The drawing under review shows one solid part. Ordinate dimensions are in mm from its lowest x, y, z. A direction names the side the tool comes from. Coordinates: 2 decimals unless noted, no trailing zeros. Order: outer loops, then holes, each group sorted by start corner. A loop starts at its lowest first (then second) coordinate and runs counter-clockwise, first axis right, second up. Notation, with made-up numbers: M 41,73.5 L 92,73.5 A35 ccw 92,105.5 Z; hole C -23.5,-38.75 d8. An arc over 180 degrees is marked long. Answer as a JSON object with one key per item and string values.
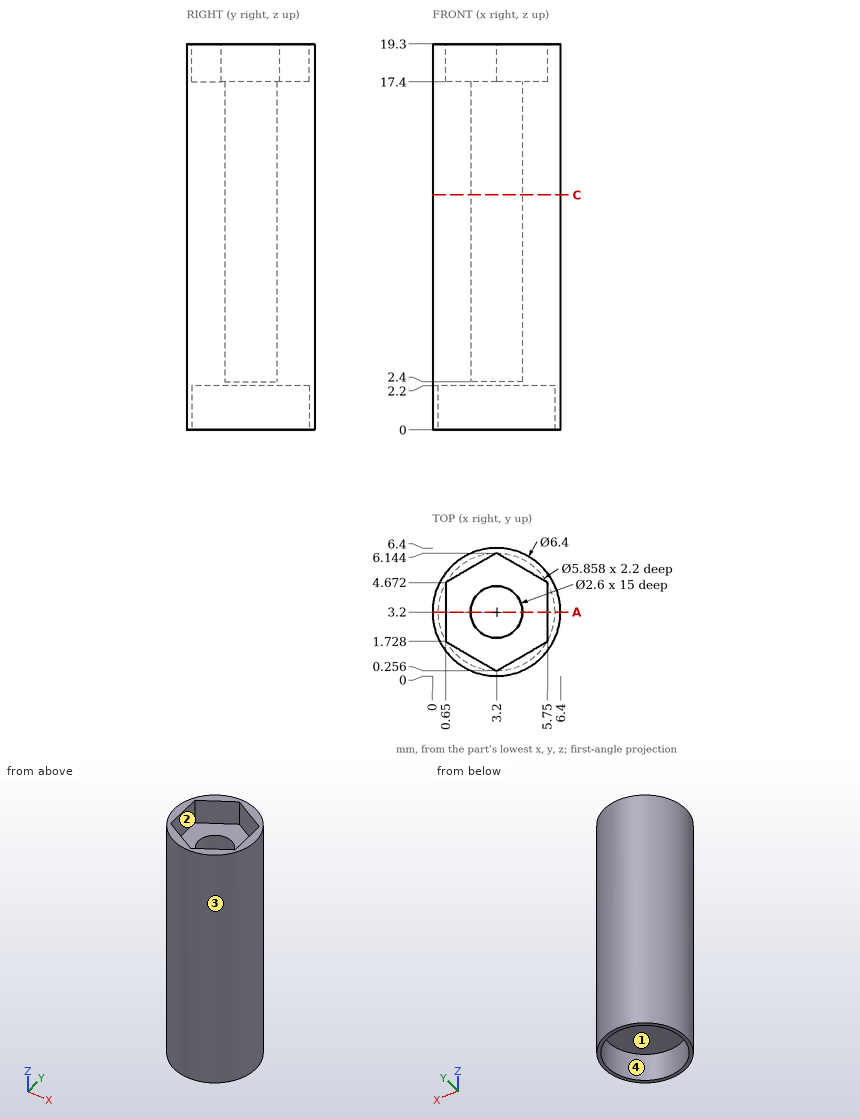
1) To check wall thickness, follow L1, parallel to Y at x = 3.2, z = 14; L2, parallel to Y at x = 3.2, z = 1.45; L3, parallel to Z at x = 4.25, y = 0.75. State the ranges of each line that lie inside material, in increasing order.
Taken from the geometry:
{"L1": "y = 0 to 1.9, 4.5 to 6.4", "L2": "y = 0 to 0.27, 6.13 to 6.4", "L3": "z = 2.2 to 19.3"}
2) Tool access review of the marked faces 1 and 2: name each direction out of +Z, -Z, +X, -X, +Y, -Y from which nothing blocks a thin tool from reaching the whole face with its end or side.
Taken from the geometry:
{"face 1": "-Z", "face 2": "+Z"}
3) Insertion check: pin 1 Ø2 at (x, z) = (3.5, 8) entering from -Y; pin 2 Ø3.5 at (x, y) = (3.2, 3.2) entering from +Z; pin 3 Ø1.8 at (x, y) = (3, 4) entering from -Z; pin 4 Ø2.5 at (x, y) = (3.2, 3.2) entering from +Z. Each pin has a flat end and moves straight along its axis. Give the tip position at first contact, or say it passes through.
Taken from the geometry:
{"pin 1": "stops at y = 0", "pin 2": "stops at z = 17.4", "pin 3": "stops at z = 2.2", "pin 4": "stops at z = 2.4"}
4) Add section A-A (y = 3.2). State the section outline as (x, z) points.
Taken from the geometry:
{"outline": "M 0,0 L 0.27,0 L 0.27,2.2 L 6.13,2.2 L 6.13,0 L 6.4,0 L 6.4,19.3 L 5.75,19.3 L 5.75,17.4 L 4.5,17.4 L 4.5,2.4 L 1.9,2.4 L 1.9,17.4 L 0.65,17.4 L 0.65,19.3 L 0,19.3 Z"}
5) Mouldability with a two-part tool opening along X and no side actions: class the marked faces 3 and 4 as released by +X, released by -X, zero draft, split by the parting line, or undercut.
Taken from the geometry:
{"face 3": "split by the parting line", "face 4": "undercut"}
6) Add section C-C (z = 11.75). State the section outline as (x, y) points.
Taken from the geometry:
{"outline": "C 3.2,3.2 d6.4; hole C 3.2,3.2 d2.6"}
